Work out the finished part from the listing and answer in its coordinate system (mm). A direction names the side the tool comes from. Coordinates: 2 decimals unless noted, no trailing zeros. Write each loop counter-clockwise with the first axis right and the second up, starting at its lowest first coordinate (ties: lowest second). Pieces come first, ordered by that corner, then holes. Notation, with made-up numbers: (-10.5, 14) - (36.5, 14) arc R25 cw to (36.5, 48) - close; hole circle Ø7 at (59, 6.5). An arc over 180 degrees is marked (long way). One line per item, written item: value.
```python
from build123d import *

# Parameters (mm, degrees)
SKETCH_1_W          = 20
SKETCH_1_H          = 100
EXTRUDE_1_DEPTH     = 10
SKETCH_2_W          = 20
SKETCH_2_H          = 20
EXTRUDE_2_DEPTH     = 15
SKETCH_3_R          = 3
CUT_EXTRUDE_1_DEPTH = 106
SKETCH_4_R          = 5
CUT_EXTRUDE_2_DEPTH = 15
SKETCH_5_W          = 20
SKETCH_5_H          = 0.5
CUT_EXTRUDE_3_DEPTH = 0.5


with BuildPart() as part:
    # 草图1 → 凸台-拉伸1 (new body)
    with BuildSketch(Plane.XY):
        with Locations((10, -50)):
            Rectangle(SKETCH_1_W, SKETCH_1_H)
    extrude(amount=EXTRUDE_1_DEPTH)

    # 草图2 → 凸台-拉伸2 (add)
    with BuildSketch(Plane(origin=(0, 0, 0), x_dir=(-1, 0, 0), z_dir=(0, 0, -1))):
        with Locations((-10, -10)):
            Rectangle(SKETCH_2_W, SKETCH_2_H)
        with Locations((-10, -90)):
            Rectangle(SKETCH_2_W, SKETCH_2_H)
    extrude(amount=EXTRUDE_2_DEPTH)

    # 草图3 → 切除-拉伸1 (cut, through all)
    with BuildSketch(Plane(origin=(0, 0, -15), x_dir=(-1, 0, 0), z_dir=(0, 0, -1))):
        with Locations((-10, -10)):
            Circle(SKETCH_3_R)
        with Locations((-10, -90)):
            Circle(SKETCH_3_R)
    extrude(amount=-CUT_EXTRUDE_1_DEPTH, mode=Mode.SUBTRACT)

    # 草图4 → 切除-拉伸2 (cut)
    with BuildSketch(Plane.XY.offset(10)):
        with Locations((10, -10)):
            Circle(SKETCH_4_R)
        with Locations((10, -90)):
            Circle(SKETCH_4_R)
    extrude(amount=-CUT_EXTRUDE_2_DEPTH, mode=Mode.SUBTRACT)

    # 草图5 → 切除-拉伸3 (cut)
    with BuildSketch(Plane.XY.offset(10)):
        with Locations((10, -79.75)):
            Rectangle(SKETCH_5_W, SKETCH_5_H)
        with Locations((10, -59.25)):
            Rectangle(SKETCH_5_W, SKETCH_5_H)
        with Locations((10, -40.25)):
            Rectangle(SKETCH_5_W, SKETCH_5_H)
        with Locations((10, -20.25)):
            Rectangle(SKETCH_5_W, SKETCH_5_H)
    extrude(amount=-CUT_EXTRUDE_3_DEPTH, mode=Mode.SUBTRACT)


solid = part.part
```
Item 1: Given pin 1 (7 mm diameter, centred on x = 10, y = -10, fed in from +Z); pin 2 (10 mm diameter, centred on x = 13.5, y = -53.5, fed in from -Z), each flat-ended and moving along its own axis, determine where each tip first touches the part or whether it passes through.
Evaluation:
pin 1: stops at z = -5
pin 2: stops at z = 0
Item 2: Consider probe 1 along Y at (x, z) = (10, -12.5); probe 2 along Y at (x, z) = (10, 1.75); probe 3 along Y at (x, z) = (3.75, -11.5). Determine where each line is inside the solid, lowest interval first.
Evaluation:
probe 1: y = -100 to -93, -87 to -80, -20 to -13, -7 to 0
probe 2: y = -100 to -95, -85 to -15, -5 to 0
probe 3: y = -100 to -80, -20 to 0
Item 3: Which of the six approach directions +Z, -Z, +X, -X, +Y, -Y give full straight-line access (tool end or side, diameter ignored) to faces 4 (the face through (10, -20, -7)), 5 (the face through (8, -5, 10)), 6 (the face through (13.3, -9.9, -5))?
Evaluation:
face 4: -Z, +X, -X
face 5: +Z, +X, -X, +Y, -Y
face 6: +Z
Item 4: Section A-A, the plane y = -90 is taken. Determine the outline of the cut face in (x, z).
Evaluation:
outline: (0, -15) - (7, -15) - (7, -5) - (5, -5) - (5, 10) - (0, 10) - close; (13, -15) - (20, -15) - (20, 10) - (15, 10) - (15, -5) - (13, -5) - close
Item 5: Determine the mould class of faces 1 (the face through (10, -80, -7)), 2 (the face through (20, -50.7, 0.5)), 3 (the face through (14.77, -8.5, 2.61)) for opening direction X: +X half, -X half, draft (parallel to the pull), parting line (faces both ways), or undercut.
Evaluation:
face 1: draft
face 2: +X half
face 3: undercut
Item 6: Section D-D, the plane z = 4.5 is taken. Determine the outline of the cut face in (x, y), then the cut area to 3 significant figures.
Evaluation:
outline: (0, -100) - (20, -100) - (20, 0) - (0, 0) - close; hole circle Ø10 at (10, -90); hole circle Ø10 at (10, -10)
area: 1,840 mm2
Item 7: Section B-B, the plane z = -9.5 is taken. Determine the outline of the cut face in (x, y), then the cut area to 3 significant figures.
Evaluation:
outline: (0, -100) - (20, -100) - (20, -80) - (0, -80) - close; (0, -20) - (20, -20) - (20, 0) - (0, 0) - close; hole circle Ø6 at (10, -90); hole circle Ø6 at (10, -10)
area: 743 mm2
